For this review, use the dimensioned drawing (mm, ordinates from the lowest corner) and the shaded views. Give positions to 0.01 mm unless a question says otherwise; leave off trailing zeros. Order: outer loops, then holes, each group sorted by start corner. A loop starts at its lowest first (then second) coordinate and runs counter-clockwise, first axis right, second up. Notation, with made-up numbers: M 1.5,-32 L 13.5,-32 A16 cw 13.5,-13 Z; hole C -24,16.5 d6. An arc over 180 degrees is marked long. One line per question, with ' | ' between items. Start each with the question number.
1. Wall thickness on L1, parallel to Y at x = 5.5, z = 8.5; L2, parallel to Z at x = 1.5, y = 5.75 (1 decimal); L3, parallel to X at y = 1.75, z = 5: over which ranges is each line inside the solid? List them lowest first.
2. We need section C-C on x = 3.75. Write out the cut boundary in (y, z) (1 decimal).
3. We need section A-A on x = 1.25. Write out the cut boundary in (y, z) (1 decimal).
4. We need section B-B on z = 7.25. Write out the cut boundary in (x, y) (1 decimal), then the cut area to 3 significant figures.
5. Insertion check: P1, Ø1.5, axis at y = 3, z = 2.5, coming from the -X side (1 decimal). The pin has a flat end and moves straight along its axis. Give the tip position at first contact, or say it passes through.
6. The part is to be moulded in two halves that separate along Z. For the marked faces 1, 2 and 3, say which applies: +Z half, -Z half, draft (parallel to the pull), parting line (faces both ways), or undercut.
7. We need section D-D on y = 1.5. Write out the cut boundary in (x, z), then the cut area to 3 significant figures.
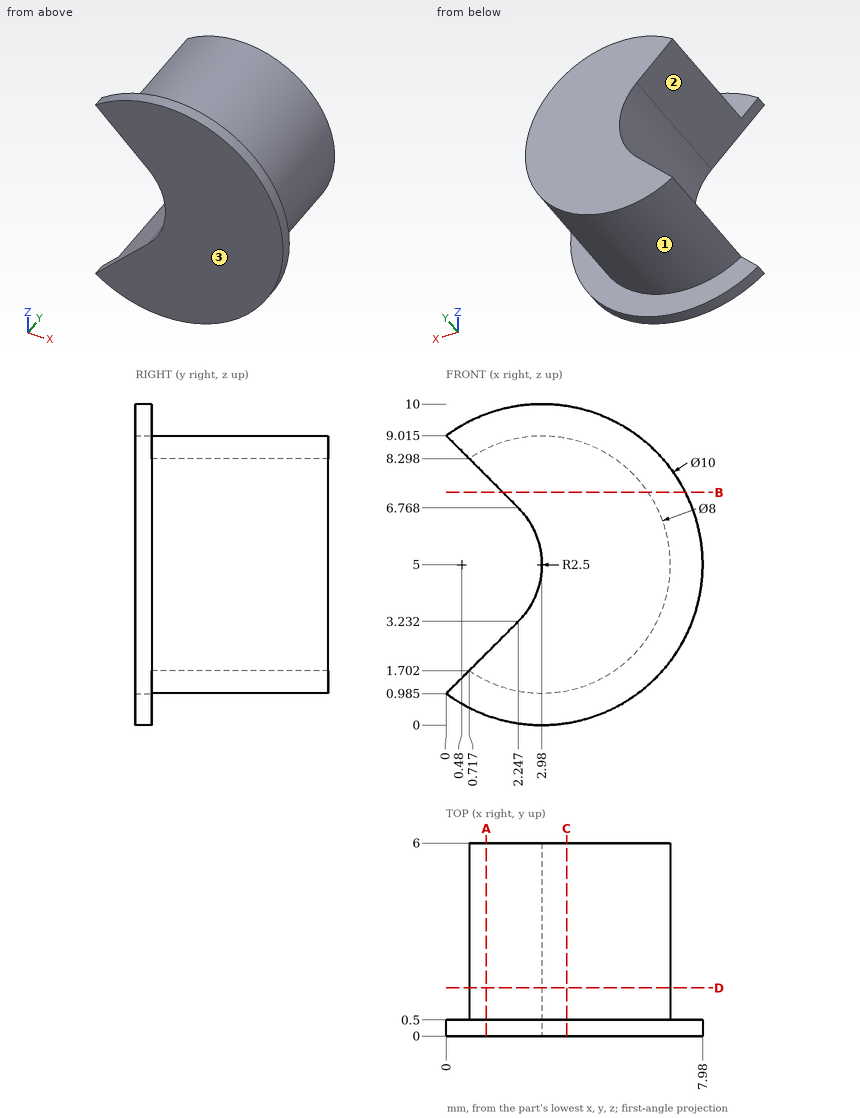
Entries:
1) L1: y = 0 to 0.5 | L2: z = 1.3 to 2.5, 7.5 to 8.7 | L3: x = 2.98 to 6.98
2) outline: M 0,0.1 L 0.5,0.1 L 0.5,1.1 L 6,1.1 L 6,8.9 L 0.5,8.9 L 0.5,9.9 L 0,9.9 Z
3) outline: M 0,0.3 L 0.5,0.3 L 0.5,1.4 L 6,1.4 L 6,2.2 L 0,2.2 Z; M 0,7.8 L 6,7.8 L 6,8.6 L 0.5,8.6 L 0.5,9.7 L 0,9.7 Z
4) outline: M 1.8,0 L 7.4,0 L 7.4,0.5 L 6.3,0.5 L 6.3,6 L 1.8,6 Z | area: 27.7 mm^2
5) P1: stops at x = 0.8
6) face 1: parting line | face 2: undercut | face 3: draft
7) outline: M 0.72,1.7 A4 ccw long 0.72,8.3 L 2.25,6.77 A2.5 cw 2.25,3.23 Z | area: 32.7 mm^2
